CAD build for the part. Positions are in the model's coordinates, mm. A direction names the side the tool comes from. Round coordinates to 2 decimals unless told otherwise and drop trailing zeros. Loops run counter-clockwise (first coordinate to the right, second up) from the corner with the lowest first, then second, coordinate; pieces in that order, holes last. Notation, with made-up numbers: (45, -18) - (98, -18) arc R27 cw to (98, 11) - close; hole circle Ø11 at (21, -30.75). An arc over 180 degrees is marked (long way). Use one line per item in the form item = value.
from build123d import *

# Parameters (mm, degrees)
SKETCH1_W           = 24
SKETCH1_H           = 15
SKETCH1_R           = 5
SKETCH1_H_2         = 2
BOSS_EXTRUDE1_DEPTH = 2
SKETCH1_3_W         = 24
SKETCH1_3_H         = 2
BOSS_EXTRUDE2_DEPTH = 30
SKETCH3_W           = 2
SKETCH3_H           = 34
BOSS_EXTRUDE3_DEPTH = 25
SKETCH4_W           = 2
SKETCH4_H           = 9.5
CUT_EXTRUDE1_DEPTH  = 25
SKETCH5_R           = 5
CUT_EXTRUDE2_DEPTH  = 64.437930135
FILLET1_R           = 10
FILLET2_R           = 2
CHAMFER1_SIZE       = 3


with BuildPart() as part:
    # Sketch1 → Boss-Extrude1 (new body)
    # profile 1 of 2: a face of its own
    with BuildSketch(Plane.XY):
        Rectangle(SKETCH1_W, SKETCH1_H)
        Circle(SKETCH1_R, mode=Mode.SUBTRACT)
    # profile 2 of 2: a face of its own
    with BuildSketch(Plane.XY):
        with Locations((0, -8.5)):
            Rectangle(SKETCH1_W, SKETCH1_H_2)
    boss_extrude1 = extrude(amount=BOSS_EXTRUDE1_DEPTH)

    # Sketch1<3> → Boss-Extrude2 (add)
    with BuildSketch(Plane.XY):
        with Locations((0, -8.5)):
            Rectangle(SKETCH1_3_W, SKETCH1_3_H)
    extrude(amount=-BOSS_EXTRUDE2_DEPTH)

    # Mirror1: Boss-Extrude1 across plane
    add(boss_extrude1.mirror(Plane(origin=(0, 0, -15), x_dir=(1, 0, 0), z_dir=(0, 0, -1))))

    # Sketch3 → Boss-Extrude3 (add)
    with BuildSketch(Plane.XZ.offset(9.5)):
        with Locations((-11, -15)):
            Rectangle(SKETCH3_W, SKETCH3_H)
        with Locations((11, -15)):
            Rectangle(SKETCH3_W, SKETCH3_H)
    extrude(amount=BOSS_EXTRUDE3_DEPTH)

    # Sketch4 → Cut-Extrude1 (cut)
    with BuildSketch(Plane.XZ.offset(34.5)):
        with Locations((-11, -27.25)):
            Rectangle(SKETCH4_W, SKETCH4_H)
        with Locations((-11, -2.75)):
            Rectangle(SKETCH4_W, SKETCH4_H)
        with Locations((11, -2.75)):
            Rectangle(SKETCH4_W, SKETCH4_H)
        with Locations((11, -27.25)):
            Rectangle(SKETCH4_W, SKETCH4_H)
    extrude(amount=-CUT_EXTRUDE1_DEPTH, mode=Mode.SUBTRACT)

    # Sketch5 → Cut-Extrude2 (cut)
    with BuildSketch(Plane(origin=(12, 0, 0), x_dir=(0, 0, -1), z_dir=(1, 0, 0))):
        with Locations((15, -24.5)):
            Circle(SKETCH5_R)
    extrude(amount=-CUT_EXTRUDE2_DEPTH, mode=Mode.SUBTRACT)

    # Fillet1
    # the kernel refuses this fillet: 10 mm, written as the material it adds along each edge
    with BuildSketch(Plane(origin=(12, -9.5, -7.5), x_dir=(0, 0, 1), z_dir=(-1, 0, 0)), Plane(origin=(-10, -9.5, -7.5), x_dir=(0, 0, 1), z_dir=(-1, 0, 0))) as fillet1_piece_1:
        with BuildLine():
            CenterArc((10, -9.987492178), FILLET1_R, 92.865983983, 87.134016017)
            Line((0, -9.987492178), (-0.2, -9.987492178))
            Line((-0.2, -9.987492178), (-0.2, 0))
            Line((-0.2, 0), (0, 0.2))
            ThreePointArc((0, 0.2), (4.75, 0.2), (9.49, 0.199749844))
            Line((9.49, 0.199749844), (9.5, 0))
        make_face()
    extrude(amount=2)
    with BuildSketch(Plane(origin=(12, -9.5, -7.5), x_dir=(0, 0, 1), z_dir=(-1, 0, 0))) as fillet1_piece_2_section:
        with BuildLine():
            CenterArc((10, -9.987492178), FILLET1_R, 92.865983983, 87.134016017)
            Line((0, -9.987492178), (-0.2, -9.987492178))
            Line((-0.2, -9.987492178), (-0.2, 0))
            Line((-0.2, 0), (0, 0.2))
            ThreePointArc((0, 0.2), (4.75, 0.2), (9.49, 0.199749844))
            Line((9.49, 0.199749844), (9.5, 0))
        make_face()
    fillet1_piece_2 = extrude(amount=26.968730444, mode=Mode.PRIVATE)
    fillet1_piece_2 = split(fillet1_piece_2, bisect_by=Plane(origin=(-12, -11.774818107, -5.276261627), z_dir=(1, 0, 0)), keep=Keep.TOP, mode=Mode.PRIVATE)
    fillet1_piece_2 = split(fillet1_piece_2, bisect_by=Plane(origin=(-10, -11.774818107, -5.276261627), z_dir=(-1, 0, 0)), keep=Keep.TOP, mode=Mode.PRIVATE)
    add(fillet1_piece_2)
    with BuildSketch(Plane(origin=(12, -9.5, -22.5), x_dir=(0, 0, -1), z_dir=(-1, 0, 0)), Plane(origin=(-10, -9.5, -22.5), x_dir=(0, 0, -1), z_dir=(-1, 0, 0))) as fillet1_piece_3:
        with BuildLine():
            CenterArc((10, 9.987492178), FILLET1_R, 180, 87.134016017)
            Line((0, 9.987492178), (-0.2, 9.987492178))
            Line((-0.2, 9.987492178), (-0.2, 0))
            Line((-0.2, 0), (0, -0.2))
            ThreePointArc((0, -0.2), (4.75, -0.2), (9.49, -0.199749844))
            Line((9.49, -0.199749844), (9.5, 0))
        make_face()
    extrude(amount=2)
    with BuildSketch(Plane(origin=(12, -9.5, -22.5), x_dir=(0, 0, -1), z_dir=(-1, 0, 0))) as fillet1_piece_4_section:
        with BuildLine():
            CenterArc((10, 9.987492178), FILLET1_R, 180, 87.134016017)
            Line((0, 9.987492178), (-0.2, 9.987492178))
            Line((-0.2, 9.987492178), (-0.2, 0))
            Line((-0.2, 0), (0, -0.2))
            ThreePointArc((0, -0.2), (4.75, -0.2), (9.49, -0.199749844))
            Line((9.49, -0.199749844), (9.5, 0))
        make_face()
    fillet1_piece_4 = extrude(amount=26.968730444, mode=Mode.PRIVATE)
    fillet1_piece_4 = split(fillet1_piece_4, bisect_by=Plane(origin=(-12, -11.774818107, -24.723738373), z_dir=(1, 0, 0)), keep=Keep.TOP, mode=Mode.PRIVATE)
    fillet1_piece_4 = split(fillet1_piece_4, bisect_by=Plane(origin=(-10, -11.774818107, -24.723738373), z_dir=(-1, 0, 0)), keep=Keep.TOP, mode=Mode.PRIVATE)
    add(fillet1_piece_4)
    with BuildSketch(Plane(origin=(14.968730444, -9.5, -22.5), x_dir=(0, 0, -1), z_dir=(-1, 0, 0))) as fillet1_piece_5_section:
        with BuildLine():
            CenterArc((10, 9.987492178), FILLET1_R, 180, 87.134016017)
            Line((0, 9.987492178), (-0.2, 9.987492178))
            Line((-0.2, 9.987492178), (-0.2, 0))
            Line((-0.2, 0), (0, -0.2))
            ThreePointArc((0, -0.2), (4.75, -0.2), (9.49, -0.199749844))
            Line((9.49, -0.199749844), (9.5, 0))
        make_face()
    fillet1_piece_5 = extrude(amount=26.968730444, mode=Mode.PRIVATE)
    fillet1_piece_5 = split(fillet1_piece_5, bisect_by=Plane(origin=(12, -11.774818107, -24.723738373), z_dir=(-1, 0, 0)), keep=Keep.TOP, mode=Mode.PRIVATE)
    fillet1_piece_5 = split(fillet1_piece_5, bisect_by=Plane(origin=(10, -11.774818107, -24.723738373), z_dir=(1, 0, 0)), keep=Keep.TOP, mode=Mode.PRIVATE)
    add(fillet1_piece_5)
    with BuildSketch(Plane(origin=(14.968730444, -9.5, -7.5), x_dir=(0, 0, 1), z_dir=(-1, 0, 0))) as fillet1_piece_6_section:
        with BuildLine():
            CenterArc((10, -9.987492178), FILLET1_R, 92.865983983, 87.134016017)
            Line((0, -9.987492178), (-0.2, -9.987492178))
            Line((-0.2, -9.987492178), (-0.2, 0))
            Line((-0.2, 0), (0, 0.2))
            ThreePointArc((0, 0.2), (4.75, 0.2), (9.49, 0.199749844))
            Line((9.49, 0.199749844), (9.5, 0))
        make_face()
    fillet1_piece_6 = extrude(amount=26.968730444, mode=Mode.PRIVATE)
    fillet1_piece_6 = split(fillet1_piece_6, bisect_by=Plane(origin=(12, -11.774818107, -5.276261627), z_dir=(-1, 0, 0)), keep=Keep.TOP, mode=Mode.PRIVATE)
    fillet1_piece_6 = split(fillet1_piece_6, bisect_by=Plane(origin=(10, -11.774818107, -5.276261627), z_dir=(1, 0, 0)), keep=Keep.TOP, mode=Mode.PRIVATE)
    add(fillet1_piece_6)

    # Fillet2
    fillet2_edges = [part.edges().sort_by_distance(p)[0] for p in [
        (0, -7.5, 0),
        (0, -7.5, -30),
    ]]
    fillet(fillet2_edges, radius=FILLET2_R)

    # Chamfer1
    chamfer1_edges = [part.edges().sort_by_distance(p)[0] for p in [
        (-11, -34.5, -7.5),
        (-12, 7.5, 1),
        (12, 7.5, 1),
        (-11, -34.5, -22.5),
        (-12, 7.5, -31),
        (12, 7.5, -31),
        (11, -34.5, -22.5),
        (11, -34.5, -7.5),
    ]]
    chamfer(chamfer1_edges, length=CHAMFER1_SIZE)


solid = part.part
1) Slice it at D-D (z = -8). Write the cut outline in (x, y).
Report:
outline = (-12, -32) - (-10, -32) - (-10, -9.5) - (10, -9.5) - (10, -32) - (12, -32) - (12, -7.5) - (-12, -7.5) - close
2) Slice it at B-B (z = -12). Write the cut outline in (x, y).
Report:
outline = (-12, -34.5) - (-10, -34.5) - (-10, -28.5) - (-12, -28.5) - close; (-12, -20.5) - (-10, -20.5) - (-10, -9.5) - (10, -9.5) - (10, -20.5) - (12, -20.5) - (12, -7.5) - (-12, -7.5) - close; (10, -34.5) - (12, -34.5) - (12, -28.5) - (10, -28.5) - close
3) Tool access for faces 4 (the flat face through (-10, -19, -15)), 5 (the flat face through (-0.2, 5.4, -30)), 6 (the flat face through (-11, -26, -7.5)): list every direction of +Z, -Z, +X, -X, +Y, -Y with a clear straight run to the whole face (end or side of a thin tool).
Report:
face_4 = +Z, -Z, -Y
face_5 = +X, -X, +Y
face_6 = +Z, +X, -X, -Y
4) Drill centre lines: probe 1 along Y at (x, z) = (11.45, -15); probe 2 along Y at (x, z) = (0, 1.1); probe 3 along Z at (x, y) = (11, 0.5). Where is each one in solid material? Low to high.
Report:
probe_1 = -34.5 to -29.5, -19.5 to -7.5
probe_2 = -9.5 to -5, 5 to 7.5
probe_3 = -32 to -30, 0 to 2
5) Flat gauge pins, fed straight in: pin 1 (0.6 mm diameter, centred on x = -11.5, y = -22.5, fed in from -Z); pin 2 (9 mm diameter, centred on x = 0, y = 0, fed in from +Z); pin 3 (1.5 mm diameter, centred on x = 3, z = -5, fed in from -Y); pin 4 (1 mm diameter, centred on x = -11.5, y = -23.5, fed in from +Z). Where does each tip first touch, or does it go through?
Report:
pin_1 = -22.5
pin_2 = through
pin_3 = -9.5
pin_4 = -7.5
6) Slice it at A-A (y = -24.5). Write the cut outline in (x, z), plus the area to 3 significant figures.
Report:
outline = (-12, -22.5) - (-10, -22.5) - (-10, -20) - (-12, -20) - close; (-12, -10) - (-10, -10) - (-10, -7.5) - (-12, -7.5) - close; (10, -22.5) - (12, -22.5) - (12, -20) - (10, -20) - close; (10, -10) - (12, -10) - (12, -7.5) - (10, -7.5) - close
area = 20.0 mm^2
7) Two-plate mould, pull along X, no slides. Class faces 1 (the flat face through (12, -15, -14)), 2 (the flat face through (10, -19, -15)), 3 (the cylindrical face through (-10.986, -12.519, -4.672)): +X half, -X half, draft (parallel to the pull), parting line (faces both ways), or undercut.
Report:
face_1 = +X half
face_2 = undercut
face_3 = draft
8) Slice it at C-C (x = -0.5). Write the cut outline in (y, z), plus the area to 3 significant figures.
Report:
outline = (-9.5, -32) - (-4.97, -32) - (-4.97, -30) - (-5.5, -30) arc R2 cw to (-7.5, -28) - (-7.5, -2) arc R2 cw to (-5.5, 0) - (-4.97, 0) - (-4.97, 2) - (-9.5, 2) - close; (4.97, -32) - (7.5, -32) - (7.5, -30) - (4.97, -30) - close; (4.97, 0) - (7.5, 0) - (7.5, 2) - (4.97, 2) - close
area = 89.9 mm^2
